Geometry: see drawing. Coordinates: mm, zero at the bounding-box minimum. Give positions to 0.01 mm unless a question says otherwise; leave off trailing zeros. Order: outer loops, then holes, each group sorted by start corner. A loop starts at its lowest first (then second) coordinate and runs counter-clockwise, first axis right, second up. Notation, with made-up numbers: (55, 38) - (86, 38) arc R25 ccw to (86, 71) - close; hole circle Ø1 at (77.5, 11.5). An arc over 180 degrees is marked (long way). Write item = value, one per line. Start each with the question number.
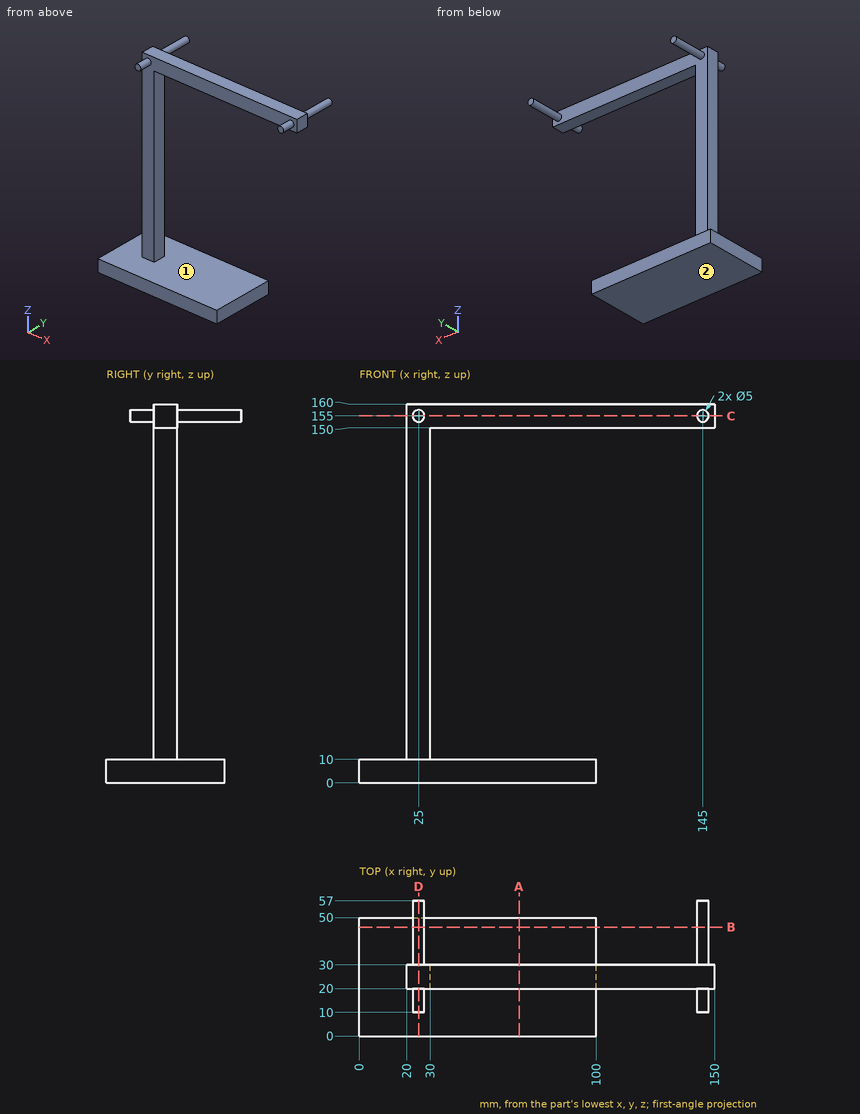
Q1. Section A-A, the plane x = 67.5. Return the cut outline in (y, z).
Q2. Section D-D, the plane x = 25. Return the cut outline in (y, z).
Q3. Material intervals for line 1 along Z through (x, y) = (98.5, 21); line 2 along Y through (x, z) = (64, 152.5); line 3 along Z through (x, y) = (68.5, 38), sorted ascending. Write a range as from..to.
Q4. Contact query for flat-ended pins moving along their axis: pin 1 (5.5 mm diameter, centred on x = 144.5, z = 156, fed in from -Y); pin 2 (11 mm diameter, centred on x = 66, y = 25, fed in from -Z); pin 3 (11 mm diameter, centred on y = 24, z = 91, fed in from -X); pin 4 (8 mm diameter, centred on x = 68, z = 6.5, fed in from +Y). Output: stop coordinate, or through.
Q5. Pull-direction query (Z, two-part tool) for the marked faces 1 and 2; classes: +Z half, -Z half, draft (parallel to the pull), parting line (faces both ways), or undercut.
Q6. Section B-B, the plane y = 46. Return the cut outline in (x, z), then the cut area to 3 significant figures.
Q7. Section C-C, the plane z = 155. Return the cut outline in (x, y), then the cut area to 3 significant figures.
The answers:
q1.outline = (0, 0) - (50, 0) - (50, 10) - (0, 10) - close; (20, 150) - (30, 150) - (30, 160) - (20, 160) - close
q2.outline = (0, 0) - (50, 0) - (50, 10) - (30, 10) - (30, 152.5) - (57, 152.5) - (57, 157.5) - (30, 157.5) - (30, 160) - (20, 160) - (20, 157.5) - (10, 157.5) - (10, 152.5) - (20, 152.5) - (20, 10) - (0, 10) - close
q3.line_1 = 0..10, 150..160
q3.line_2 = 20..30
q3.line_3 = 0..10
q4.pin_1 = 10
q4.pin_2 = 0
q4.pin_3 = 20
q4.pin_4 = 50
q5.face_1 = undercut
q5.face_2 = -Z half
q6.outline = (0, 0) - (100, 0) - (100, 10) - (0, 10) - close; circle Ø5 at (25, 155); circle Ø5 at (145, 155)
q6.area = 1,040 mm²
q7.outline = (20, 20) - (22.5, 20) - (22.5, 10) - (27.5, 10) - (27.5, 20) - (142.5, 20) - (142.5, 10) - (147.5, 10) - (147.5, 20) - (150, 20) - (150, 30) - (147.5, 30) - (147.5, 57) - (142.5, 57) - (142.5, 30) - (27.5, 30) - (27.5, 57) - (22.5, 57) - (22.5, 30) - (20, 30) - close
q7.area = 1,670 mm²
